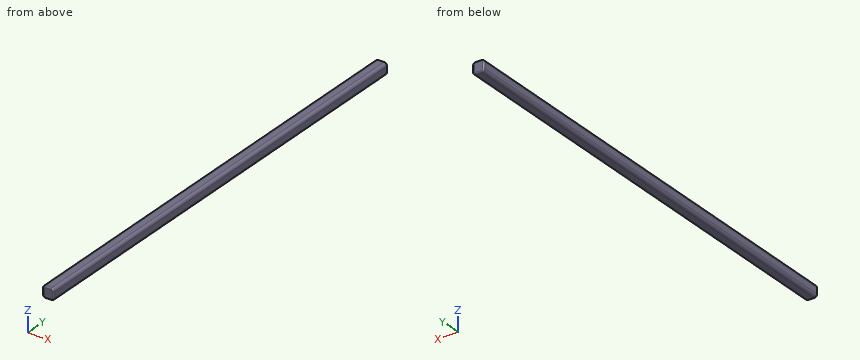
Autodesk Inventor part; units mm, degrees
ref_plane "YZ Plane" through (0, 0, 0) normal (1, 0, 0) x (0, 1, 0)
ref_plane "XZ Plane" through (0, 0, 0) normal (0, 1, 0) x (-1, 0, 0)
ref_plane "XY Plane" through (0, 0, 0) normal (0, 0, 1) x (1, 0, 0)
sketch "Sketch1" plane through (0, 0, 0) normal (0, 1, 0) x (-1, 0, 0)
  line L0 (-3.175, 3.175) -> (3.175, 3.175)
  line L1 (3.175, 3.175) -> (3.175, -3.175)
  line L2 (3.175, -3.175) -> (-3.175, -3.175)
  line L3 (-3.175, -3.175) -> (-3.175, 3.175)
  line L4 (-3.175, 3.175) -> (3.175, -3.175) construction
  line L5 (3.175, 3.175) -> (-3.175, -3.175) construction
  point P0 (0, 0)
  dimension "d0" = 6.35
  dimension "d1" = 6.35
extrude "Extrusion1" add sketch "Sketch1" along normal blind 254
fillet "Fillet1" radius 1.5875 4 edges at (3.175, 127, 3.175) (-3.175, 127, -3.175) (-3.175, 127, 3.175) (3.175, 127, -3.175)
fillet "Fillet2" radius 0.7937 16 edges at (3.175, 0, 0) (2.71, 0, -2.71) (0, 0, -3.175) (-2.71, 0, -2.71) (-3.175, 0, 0) (-2.71, 0, 2.71) (0, 0, 3.175) (2.71, 0, 2.71) (0, 254, 3.175) (-2.71, 254, 2.71) (-3.175, 254, 0) (-2.71, 254, -2.71) (0, 254, -3.175) (2.71, 254, -2.71) (3.175, 254, 0) (2.71, 254, 2.71)
properties part number "10 inch hs shaft" material "Stainless Steel"
Read the model definition and answer for the solid it produces. Units are mm, in the model's axes. Give positions to 0.01 mm unless a question says otherwise; leave off trailing zeros. Write each loop counter-clockwise with the first axis right and the second up, starting at its lowest first coordinate (ties: lowest second). Pieces come first, ordered by that corner, then holes. Notation, with made-up numbers: M 47.5,15.5 L 92.5,15.5 A6 cw 92.5,22.5 Z; hole C 12,50 d5. An arc over 180 degrees is marked long. One line per item, written item: value. Start each with the question number.
(1) Find section A-A (y = 236). Determine the outline of the cut face in (x, z) (1 decimal).
(2) A flat-ended cylindrical pin translates along its axis: pin 1 Ø1 at (x, y) = (2.5, 181) entering from +Z. Find the tip coordinate at first contact, or state that the pin passes through.
(3) Find the intervals of material crossed by line 1 (X direction, y = 73.5, z = 1.75); line 2 (Y direction, x = -2.5, z = -0.5), in increasing order.
Results below:
1. outline: M -3.2,-1.6 A1.6 ccw -1.6,-3.2 L 1.6,-3.2 A1.6 ccw 3.2,-1.6 L 3.2,1.6 A1.6 ccw 1.6,3.2 L -1.6,3.2 A1.6 ccw -3.2,1.6 Z
2. pin 1: stops at z = 3.12
3. line 1: x = -3.17 to 3.17
3. line 2: y = 0.01 to 253.99
